Design review of the part built by this model. Coordinates are the model's own, in mm. Face numbers are marked on the shaded views. A direction names the side the tool comes from. Coordinates: 2 decimals unless noted, no trailing zeros. Write each loop counter-clockwise with the first axis right and the second up, starting at its lowest first coordinate (ties: lowest second). Pieces come first, ordered by that corner, then holes.
```python
from build123d import *

# Parameters (mm, degrees)
F0_W     = 50
F0_H     = 65
F1_DEPTH = 38
F2_R     = 10
F3_T     = -2
F4_W     = 14
F4_H     = 20
F5_DEPTH = 25
F6_R     = 6


with BuildPart() as f1:
    # F0 (on Top) → F1 (new body)
    with BuildSketch(Plane.XY):
        Rectangle(F0_W, F0_H)
    extrude(amount=F1_DEPTH)

    # F2
    f2_edges = [f1.edges().sort_by_distance(p)[0] for p in [
        (0, 32.5, 38),
        (25, 32.5, 19),
        (25, 0, 38),
        (25, -32.5, 19),
        (0, -32.5, 38),
        (-25, 0, 38),
        (-25, 32.5, 19),
        (-25, -32.5, 19),
    ]]
    fillet(f2_edges, radius=F2_R)

    # F3
    f3_openings = [f1.faces().sort_by_distance(p)[0] for p in [
        (0, 0, 0),
    ]]
    offset(amount=F3_T, openings=f3_openings)

    # F4 (on face) → F5 (cut)
    with BuildSketch(Plane(origin=(0, 32.5, 0), x_dir=(-1, 0, 0), z_dir=(0, 1, 0))):
        with Locations((0, 10)):
            Rectangle(F4_W, F4_H)
    extrude(amount=-F5_DEPTH, mode=Mode.SUBTRACT)

    # F6
    f6_edges = [f1.edges().sort_by_distance(p)[0] for p in [
        (7, 31.5, 20),
        (-7, 31.5, 20),
    ]]
    fillet(f6_edges, radius=F6_R)


solid = f1.part
```
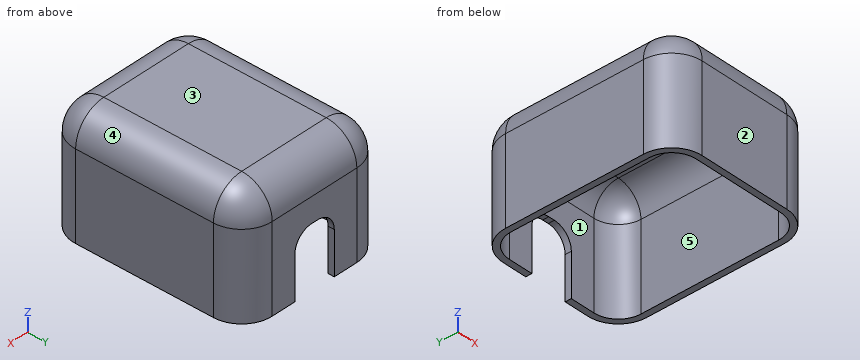
(1) Insertion check: pin 1 Ø1.6 at (x, y) = (0, 31.5) entering from -Z; pin 2 Ø12 at (x, y) = (-5.5, -21) entering from -Z; pin 3 Ø2 at (x, z) = (-14, 28.5) entering from +Y; pin 4 Ø1 at (y, z) = (31.5, 7.5) entering from +X. Each pin has a flat end and moves straight along its axis. Give the tip position at first contact, or say it passes through.
(2) Consider section C-C (x = -13.5). Give the boundary of the cut face in (y, z).
(3) Consider section D-D (z = 7). Give the boundary of the cut face in (x, y).
(4) Consider section B-B (y = 14). Give the boundary of the cut face in (x, z).
(5) Wall thickness on line 1 (X direction, y = 12, z = 12.5); line 2 (Y direction, x = -0.5, z = 27); line 3 (Y direction, x = 1, z = 34): over which ranges is each line inside the solid? List them lowest first.
(6) Consider section A-A (z = 21). Give the boundary of the cut face in (x, y).
(7) Mouldability with a two-part tool opening along X and no side actions: class the marked faces 3, 4 and 5 as +X half, -X half, draft (parallel to the pull), parting line (faces both ways), or undercut.
(8) For the marked faces 1 and 2, list the 3-axis set-ups (+Z, -Z, +X, -X, +Y, -Y) from which the entire face can be reached by the end or side of a thin tool; tool diameter is ignored.
Results:
1. pin 1: stops at z = 20
1. pin 2: stops at z = 34.61
1. pin 3: stops at y = 32.5
1. pin 4: stops at x = 20.27
2. outline: (-32.5, 0) - (-30.5, 0) - (-30.5, 28) arc R8 cw to (-22.5, 36) - (22.5, 36) arc R8 cw to (30.5, 28) - (30.5, 0) - (32.5, 0) - (32.5, 28) arc R10 ccw to (22.5, 38) - (-22.5, 38) arc R10 ccw to (-32.5, 28) - close
3. outline: (-25, -22.5) arc R10 ccw to (-15, -32.5) - (15, -32.5) arc R10 ccw to (25, -22.5) - (25, 22.5) arc R10 ccw to (15, 32.5) - (7, 32.5) - (7, 30.5) - (15, 30.5) arc R8 cw to (23, 22.5) - (23, -22.5) arc R8 cw to (15, -30.5) - (-15, -30.5) arc R8 cw to (-23, -22.5) - (-23, 22.5) arc R8 cw to (-15, 30.5) - (-7, 30.5) - (-7, 32.5) - (-15, 32.5) arc R10 ccw to (-25, 22.5) - close
4. outline: (-25, 0) - (-23, 0) - (-23, 28) arc R8 cw to (-15, 36) - (15, 36) arc R8 cw to (23, 28) - (23, 0) - (25, 0) - (25, 28) arc R10 ccw to (15, 38) - (-15, 38) arc R10 ccw to (-25, 28) - close
5. line 1: x = -25 to -23, 23 to 25
5. line 2: y = -32.5 to -30.5, 30.5 to 32.5
5. line 3: y = -30.5 to -27.79, 27.79 to 30.5
6. outline: (-25, -22.5) arc R10 ccw to (-15, -32.5) - (15, -32.5) arc R10 ccw to (25, -22.5) - (25, 22.5) arc R10 ccw to (15, 32.5) - (-15, 32.5) arc R10 ccw to (-25, 22.5) - close; hole (-23, -22.5) arc R8 ccw to (-15, -30.5) - (15, -30.5) arc R8 ccw to (23, -22.5) - (23, 22.5) arc R8 ccw to (15, 30.5) - (-15, 30.5) arc R8 ccw to (-23, 22.5) - close
7. face 3: draft
7. face 4: +X half
7. face 5: undercut
8. face 1: -Z
8. face 2: +Z, -Z, +X, -X, -Y
